Could you check a few things on this model? Use its own coordinates, in mm. Round coordinates to 2 decimals unless told otherwise and drop trailing zeros. Loops run counter-clockwise (first coordinate to the right, second up) from the corner with the lowest first, then second, coordinate; pieces in that order, holes last. Notation, with made-up numbers: (-12.5, 79.25) -> (27.5, 79.25) arc R17 ccw to (27.5, 92.25) -> close; hole circle Ø11 at (-9, 25). An arc over 180 degrees is marked (long way). Write each question's results on one line, items separated by ' | '. Start each with the question number.
1) If I drill on probe 1 along X at (y, z) = (0.05, 23); probe 2 along Z at (x, y) = (28.5, 0.05), over which ranges is the centre line in solid material (lowest first)?
2) Imagine slicing it at B-B, the plane z = -1.5. Give the number of separate pieces and of enclosed holes in the cut face, plus the area to 3 significant figures.
3) For P1, Ø7, axis at x = 0, z = 0, coming from the -Y side; P2, Ø3, axis at x = 15, z = 7, coming from the -Y side, each with a flat end and sliding along its axis, tell me the tip position at first contact or that it passes through.
4) Imagine slicing it at A-A, the plane z = -19.5. List the corners of the cut face in (x, y) for me, plus the area to 3 significant figures.
from build123d import *

# Parameters (mm, degrees)
SKETCH1_R           = 32
SKETCH1_R_2         = 6
BOSS_EXTRUDE1_DEPTH = 0.3


with BuildPart() as part:
    # Sketch1 → Boss-Extrude1 (new body)
    with BuildSketch(Plane(origin=(0, 0, 0), x_dir=(1, 0, 0), z_dir=(0, 1, 0))):
        Circle(SKETCH1_R)
        Circle(SKETCH1_R_2, mode=Mode.SUBTRACT)
        with BuildLine():
            ThreePointArc((0, 26.5), (-26.097405455, 4.601676708), (-9.063533798, -24.901854451))
            ThreePointArc((-9.063533798, -24.901854451), (-8.422677416, -24.603018212), (-8.721513655, -23.96216183))
            ThreePointArc((-8.721513655, -23.96216183), (-25.112597702, 4.428028531), (0, 25.5))
            ThreePointArc((0, 25.5), (0.5, 26), (0, 26.5))
        make_face(mode=Mode.SUBTRACT)
        with BuildLine():
            ThreePointArc((22.5, 0), (3.907083998, 22.158174443), (-21.143083968, 7.695453225))
            ThreePointArc((-21.143083968, 7.695453225), (-20.844247729, 7.054596843), (-20.203391347, 7.353433082))
            ThreePointArc((-20.203391347, 7.353433082), (3.73343582, 21.17336669), (21.5, 0))
            ThreePointArc((21.5, 0), (22, -0.5), (22.5, 0))
        make_face(mode=Mode.SUBTRACT)
        with BuildLine():
            ThreePointArc((0, -26.5), (26.097405455, -4.601676708), (9.063533798, 24.901854451))
            ThreePointArc((9.063533798, 24.901854451), (8.422677416, 24.603018212), (8.721513655, 23.96216183))
            ThreePointArc((8.721513655, 23.96216183), (25.112597702, -4.428028531), (0, -25.5))
            ThreePointArc((0, -25.5), (-0.5, -26), (0, -26.5))
        make_face(mode=Mode.SUBTRACT)
        with BuildLine():
            ThreePointArc((0, 18.5), (-18.218943431, 3.212491287), (-6.327372652, -17.384313485))
            ThreePointArc((-6.327372652, -17.384313485), (-5.686516269, -17.085477246), (-5.985352508, -16.444620864))
            ThreePointArc((-5.985352508, -16.444620864), (-17.234135678, 3.038843109), (0, 17.5))
            ThreePointArc((0, 17.5), (0.5, 18), (0, 18.5))
        make_face(mode=Mode.SUBTRACT)
        with BuildLine():
            ThreePointArc((14.5, 0), (2.517898576, 14.279712419), (-13.625543001, 4.959292078))
            ThreePointArc((-13.625543001, 4.959292078), (-13.326706763, 4.318435696), (-12.685850381, 4.617271935))
            ThreePointArc((-12.685850381, 4.617271935), (2.344250399, 13.294904666), (13.5, 0))
            ThreePointArc((13.5, 0), (14, -0.5), (14.5, 0))
        make_face(mode=Mode.SUBTRACT)
        with BuildLine():
            ThreePointArc((0, -18.5), (18.218943431, -3.212491287), (6.327372652, 17.384313485))
            ThreePointArc((6.327372652, 17.384313485), (5.686516269, 17.085477246), (5.985352508, 16.444620864))
            ThreePointArc((5.985352508, 16.444620864), (17.234135678, -3.038843109), (0, -17.5))
            ThreePointArc((0, -17.5), (-0.5, -18), (0, -18.5))
        make_face(mode=Mode.SUBTRACT)
        with BuildLine():
            ThreePointArc((0, 10.5), (-10.340481407, 1.823305866), (-3.591211505, -9.866772518))
            ThreePointArc((-3.591211505, -9.866772518), (-2.950355123, -9.56793628), (-3.249191362, -8.927079897))
            ThreePointArc((-3.249191362, -8.927079897), (-9.355673654, 1.649657688), (0, 9.5))
            ThreePointArc((0, 9.5), (0.5, 10), (0, 10.5))
        make_face(mode=Mode.SUBTRACT)
        with BuildLine():
            ThreePointArc((0, -10.5), (10.340481407, -1.823305866), (3.591211505, 9.866772518))
            ThreePointArc((3.591211505, 9.866772518), (2.950355123, 9.56793628), (3.249191362, 8.927079897))
            ThreePointArc((3.249191362, 8.927079897), (9.355673654, -1.649657688), (0, -9.5))
            ThreePointArc((0, -9.5), (-0.5, -10), (0, -10.5))
        make_face(mode=Mode.SUBTRACT)
        with BuildLine():
            ThreePointArc((-14.5, 0), (-2.517898576, -14.279712419), (13.625543001, -4.959292078))
            ThreePointArc((13.625543001, -4.959292078), (13.326706763, -4.318435696), (12.685850381, -4.617271935))
            ThreePointArc((12.685850381, -4.617271935), (-2.344250399, -13.294904666), (-13.5, 0))
            ThreePointArc((-13.5, 0), (-14, 0.5), (-14.5, 0))
        make_face(mode=Mode.SUBTRACT)
        with BuildLine():
            ThreePointArc((-22.5, 0), (-3.907083998, -22.158174443), (21.143083968, -7.695453225))
            ThreePointArc((21.143083968, -7.695453225), (20.844247729, -7.054596843), (20.203391347, -7.353433082))
            ThreePointArc((20.203391347, -7.353433082), (-3.73343582, -21.17336669), (-21.5, 0))
            ThreePointArc((-21.5, 0), (-22, 0.5), (-22.5, 0))
        make_face(mode=Mode.SUBTRACT)
    extrude(amount=BOSS_EXTRUDE1_DEPTH)


solid = part.part
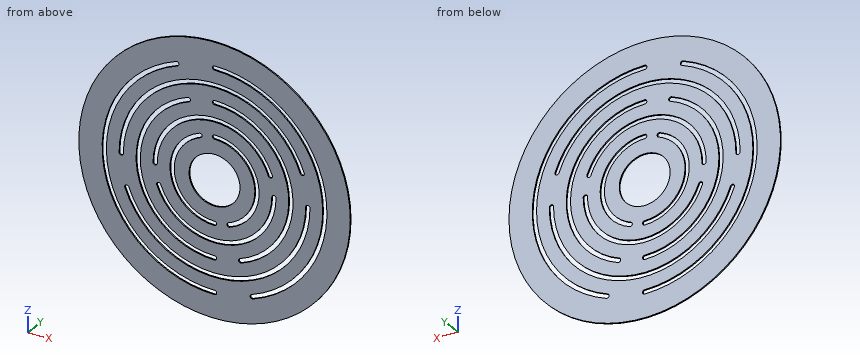
Checked values:
1) probe 1: -22.25 to -13.16, -11.01 to 11.01, 13.16 to 22.25 | probe 2: -14.55 to 14.55
2) separate pieces: 10 | enclosed holes: 0 | area: 13.3 mm^2
3) P1: through | P2: y = 0
4) outline: (-25.37, 0) -> (-17.94, 0) -> (-17.94, 0.3) -> (-25.37, 0.3) -> close; (-16.43, 0) -> (-11.22, 0) -> (-11.22, 0.3) -> (-16.43, 0.3) -> close; (-9.06, 0) -> (9.06, 0) -> (9.06, 0.3) -> (-9.06, 0.3) -> close; (11.22, 0) -> (16.43, 0) -> (16.43, 0.3) -> (11.22, 0.3) -> close; (17.94, 0) -> (25.37, 0) -> (25.37, 0.3) -> (17.94, 0.3) -> close | area: 13.0 mm^2
